Source: CAD feature listing. Evaluate the final solid. Frame: model axes, mm. Coordinates: 2 decimals unless noted, no trailing zeros. Order: outer loops, then holes, each group sorted by start corner. A loop starts at its lowest first (then second) coordinate and runs counter-clockwise, first axis right, second up.
Item 1: Section C-C on x = 31. Return the cut outline in (y, z), then the cut area to 3 significant figures.
Item 2: Section B-B on z = -9.5. Return the cut outline in (x, y), then the cut area to 3 significant figures.
Item 3: Section D-D on y = 25.5. Return the cut outline in (x, z), then the cut area to 3 significant figures.
Item 4: Ray query, line 1 (X direction, y = 31, z = -15.5); line 2 (Z direction, x = 18.5, y = -37.5); line 3 (X direction, y = 11.5, z = -37). Return the intervals inside material, ascending.
Item 5: Section A-A on y = -10. Return the cut outline in (x, z).
Item 6: Contact query for flat-ended pins moving along their axis: P1, Ø4, axis at y = -37.5, z = -51, coming from the +X side; P2, Ø12, axis at x = 42.5, y = -11, coming from the +Z side; P3, Ø5, axis at y = -25.5, z = 5.5, coming from the +X side. Output: stop coordinate, or through.
from build123d import *

# Parameters (mm, degrees)
OBR_T1_ANGLE               = 180
WYTNIJ_WYCI_GNI_CIE6_DEPTH = 172.464281995
WYTNIJ_WYCI_GNI_CIE7_DEPTH = 166.271168412


with BuildPart() as part:
    # Szkic1 → Obrót1 (revolve)
    with BuildSketch(Plane(origin=(0, 0, 0), x_dir=(0, 0, -1), z_dir=(1, 0, 0))):
        with BuildLine():
            Line((0, -55), (0, 55))
            Line((0, 55), (-75, 55))
            ThreePointArc((-75, 55), (-93.005376189, 0), (-75, -55))
            Line((-75, -55), (0, -55))
        make_face()
    revolve(axis=Axis((0, -55, 0), (0, 1, 0)), revolution_arc=OBR_T1_ANGLE)

    # Szkic2 → Wytnij-wyciągnięcie6 (cut, through all)
    with BuildSketch(Plane.XZ.offset(55)):
        with BuildLine():
            Line((-50.140376582, 0), (-26.065901524, 0))
            Line((-26.065901524, 0), (-26.065901524, 75))
            Line((-26.065901524, 75), (0, 75))
            ThreePointArc((0, 75), (6.164498497, 74.746230395), (12.287280664, 73.986638888))
            ThreePointArc((12.287280664, 73.986638888), (66.513138224, 34.655482158), (67.67766953, -32.32233047))
            Line((67.67766953, -32.32233047), (87.353699516, -51.998360457))
            Line((87.353699516, -51.998360457), (99.71705874, -51.998360457))
            Line((99.71705874, -51.998360457), (99.71705874, 112.393065192))
            Line((99.71705874, 112.393065192), (-50.140376582, 112.393065192))
            Line((-50.140376582, 112.393065192), (-50.140376582, 0))
        make_face()
    extrude(amount=-WYTNIJ_WYCI_GNI_CIE6_DEPTH, mode=Mode.SUBTRACT)

    # Szkic6 → Wytnij-wyciągnięcie7 (cut, through all)
    with BuildSketch(Plane.XZ.offset(55)):
        with BuildLine():
            ThreePointArc((67.67766953, -32.32233047), (63.439635817, 40.00515726), (0, 75))
            Line((0, 75), (0, 0))
            Line((0, 0), (17.67766953, 17.67766953))
            Line((17.67766953, 17.67766953), (67.67766953, -32.32233047))
        make_face()
    extrude(amount=-WYTNIJ_WYCI_GNI_CIE7_DEPTH, mode=Mode.SUBTRACT)


solid = part.part
Answer list:
1. outline: (-55, -68.29) arc R87.69 ccw to (55, -68.29) - (55, 4.36) - (-55, 4.36) - close
1. area: 9,450 mm2
2. outline: (0, -55) - (44.86, -55) - (44.86, 55) - (0, 55) - close
2. area: 4,930 mm2
3. outline: (0, -89.44) arc R89.44 ccw to (78.4, -43.05) - (17.68, 17.68) - (0, 0) - close
3. area: 5,350 mm2
4. line 1: x = 0 to 50.86
4. line 2: z = -83.08 to 16.86
4. line 3: x = 0 to 72.36
5. outline: (0, -92.47) arc R92.47 ccw to (80.63, -45.27) - (17.68, 17.68) - (0, 0) - close
6. P1: stops at x = 69.94
6. P2: stops at z = -1.14
6. P3: stops at x = 32.36
